from build123d import *

# Parameters (mm, degrees)
SKETCH1_W = 2.6
SKETCH1_H = 17.5


with BuildPart() as part:
    # Sketch1 → Revolve1 (revolve)
    with BuildSketch(Plane(origin=(0, 0, 0), x_dir=(1, 0, 0), z_dir=(0, 1, 0))):
        with Locations((-1.3, 0)):
            Rectangle(SKETCH1_W, SKETCH1_H)
    revolve(axis=Axis((0, 0, -13.659521107), (0, 0, 1)))

    # Sketch2 → Revolve2 (revolve)
    with BuildSketch(Plane(origin=(0, 0, 0), x_dir=(1, 0, 0), z_dir=(0, 1, 0))):
        Polygon((-2.6, -7.75), (-3.6, -8.75), (-2.6, -8.75), align=None)
    revolve2 = revolve(axis=Axis((0, 0, -14.722770412), (0, 0, 1)))

    # Mirror1: Revolve2 across plane
    add(revolve2.mirror(Plane.XY))


solid = part.part
Source: CAD feature listing. Evaluate the final solid. Frame: model axes, mm. Round coordinates to 2 decimals unless told otherwise and drop trailing zeros. Loops run counter-clockwise (first coordinate to the right, second up) from the corner with the lowest first, then second, coordinate; pieces in that order, holes last. Notation, with made-up numbers: (24.5, 80) - (46.5, 80) arc R25 cw to (46.5, 104) - close; hole circle Ø2 at (4.25, 77). An arc over 180 degrees is marked (long way). Write item = value, one per line. Start each with the question number.
(1) Ray query, line 1 along Z through (x, y) = (1.75, -2.25); line 2 along Y through (x, z) = (0, -3.75); line 3 along Z through (x, y) = (-2.25, -2.5). Return the intervals inside material, ascending. Write a range as from..to.
(2) Section query A-A, the plane y = 0. Output: boundary loops of the cut face in (x, z), plus the area to 3 significant figures.
(3) Pin query (flat end, axial travel): pin 1 (1.5 mm diameter, centred on y = 1.5, z = -0.5, fed in from -X); pin 2 (1 mm diameter, centred on x = 2, z = 0, fed in from +Y); pin 3 (1 mm diameter, centred on y = 2.5, z = -4.5, fed in from +X). Return the tip coordinate at first contact, or that it passes through.
(4) Pull-direction query (Z, two-part tool) for faces 1 (the face through (0, 0, 8.75)), 2 (the face through (0.338, -2.578, -0.109)), 3 (the face through (0, 0, -8.75)); classes: +Z half, -Z half, draft (parallel to the pull), parting line (faces both ways), or undercut.
(5) Section query C-C, the plane z = 1.5. Output: boundary loops of the cut face in (x, y).
Conclusion:
q1.line_1 = -8.75..-8, 8..8.75
q1.line_2 = -2.6..2.6
q1.line_3 = -8.75..-8.51, 8.51..8.75
q2.outline = (-3.6, -8.75) - (3.6, -8.75) - (2.6, -7.75) - (2.6, 7.75) - (3.6, 8.75) - (-3.6, 8.75) - (-2.6, 7.75) - (-2.6, -7.75) - close
q2.area = 93.0 mm2
q3.pin_1 = -2.49
q3.pin_2 = 2.12
q3.pin_3 = 1.66
q4.face_1 = +Z half
q4.face_2 = undercut
q4.face_3 = -Z half
q5.outline = circle Ø5.2 at (0, 0)
